Autodesk Inventor part; units mm, degrees
ref_plane "YZ Plane" through (0, 0, 0) normal (1, 0, 0) x (0, 1, 0)
ref_plane "XZ Plane" through (0, 0, 0) normal (0, 1, 0) x (-1, 0, 0)
ref_plane "XY Plane" through (0, 0, 0) normal (0, 0, 1) x (1, 0, 0)
sketch "Sketch1" plane through (0, 0, 0) normal (0, 0, 1) x (1, 0, 0)
  circle A0 centre (0, 0) radius 1.6
  line L0 (9.815, 0) -> (4.9075, -8.5)
  line L1 (4.9075, -8.5) -> (-4.9075, -8.5)
  line L2 (-4.9075, -8.5) -> (-9.815, 0)
  line L3 (-9.815, 0) -> (-4.9075, 8.5)
  line L4 (-4.9075, 8.5) -> (4.9075, 8.5)
  line L5 (4.9075, 8.5) -> (9.815, 0)
  circle A1 centre (0, 0) radius 9.815
  point P0 (-9.815, 0)
  point P1 (-9.815, 0)
  dimension "d0" = 3.2
  dimension "d1" = 17
extrude "Extrusion1" add sketch "Sketch1" along normal blind 4
sketch "Sketch2" plane through (0, 0, 4) normal (0, 0, 1) x (1, 0, 0)
  circle A0 centre (0, 0) radius 8
  dimension "d4" = 16
extrude "Extrusion2" add sketch "Sketch2" along normal blind 2
sketch "Sketch3" plane through (0, 0, 6) normal (0, 0, 1) x (1, 0, 0)
  circle A0 centre (0, 0) radius 6
  dimension "d7" = 12
extrude "Extrusion3" add sketch "Sketch3" along normal blind 6
thread "Thread1"
sketch "Sketch4" plane through (0, 0, 12) normal (0, 0, 1) x (1, 0, 0)
  circle A0 centre (0, 0) radius 6
hole "Hole1" at (0, 0, 12) direction (0, 0, -1) diameter 9 depth 8
fillet "Fillet1" radius 1 2 edges at (4.9075, 8.5, 0) (4.9075, 8.5, 4)
sketch "Sketch5" plane through (0, 0, 0) normal (0, 0, -1) x (-1, 0, 0)
  circle A0 centre (0, 0) radius 1.6
  circle A1 centre (0, 0) radius 9.815
  line L0 (9.815, 0) -> (4.9075, -8.5)
  line L1 (4.9075, -8.5) -> (-4.9075, -8.5)
  line L2 (-4.9075, -8.5) -> (-9.815, 0)
  line L3 (-9.815, 0) -> (-4.9075, 8.5)
  line L4 (-4.9075, 8.5) -> (4.9075, 8.5)
  line L5 (4.9075, 8.5) -> (9.815, 0)
  point P0 (-9.815, 0)
  point P1 (-9.815, 0)
extrude "Extrusion4" cut sketch "Sketch5" against normal blind 5 contours L5 A1 | A1 L0 | L4 A1 | A1 L1 | L3 A1 | A1 L2
properties part number "fix-screw"
Source: CAD feature listing. Evaluate the final solid. Frame: model axes, mm. A direction names the side the tool comes from. Round coordinates to 2 decimals unless told otherwise and drop trailing zeros. Loops run counter-clockwise (first coordinate to the right, second up) from the corner with the lowest first, then second, coordinate; pieces in that order, holes last. Notation, with made-up numbers: M 62.25,53.25 L 79.25,53.25 A24 ccw 79.25,79.25 Z; hole C 71.5,-15 d4. An arc over 180 degrees is marked long. Use a Markdown table: item, result. Add a question column.
1. Cut plane C-C, the plane y = -3.5. Output: boundary loops of the cut face in (x, z).
2. Ray query, line 1 along Y through (x, z) = (0, 3.2); line 2 along Y through (x, z) = (0, 7.5); line 3 along Z through (x, y) = (-3.75, -7). Return the intervals inside material, ascending. Write a range as [from, to].
3. Set-up query: faces 4 (the cylindrical face through (-6, 0, 9)), 5 (the flat face through (7.327, -4.31, 1.972)). Return all of +Z, -Z, +X, -X, +Y, -Y with unobstructed straight access to the full face (end or side cutting, diameter ignored); none if empty.
4. Contact query for flat-ended pins moving along their axis: pin 1 (7 mm diameter, centred on x = -1.5, y = 0, fed in from +Z); pin 2 (6 mm diameter, centred on y = 3.5, z = 6, fed in from -X); pin 3 (1 mm diameter, centred on y = 4.5, z = 5.5, fed in from -X); pin 4 (1 mm diameter, centred on x = -1.5, z = 8.5, fed in from +Y). Output: stop coordinate, or through.
5. Cut plane A-A, the plane x = 0. Output: boundary loops of the cut face in (y, z), and give its area (3 significant figures).
6. Pull-direction query (Y, two-part tool) for faces 1 (the flat face through (-2, 6, 6)), 2 (the flat face through (2, 0, 4)), 3 (the cylindrical face through (-1.73, 7.81, 4.99)); classes: +Y half, -Y half, draft (parallel to the pull), parting line (faces both ways), or undercut.
7. Cut plane D-D, the plane z = 9.75. Output: boundary loops of the cut face in (x, y).
8. Cut plane B-B, the plane z = 3.5. Output: boundary loops of the cut face in (x, y), and give its area (3 significant figures).
Solution:
| question | item | result |
|---|---|---|
| 1 | outline | M -7.79,0 L 7.79,0 L 7.79,4 L 7.19,4 L 7.19,6 L 4.87,6 L 4.87,12 L 2.83,12 L 2.83,4 L -2.83,4 L -2.83,12 L -4.87,12 L -4.87,6 L -7.19,6 L -7.19,4 L -7.79,4 Z |
| 2 | line 1 | y = [-8.5, -1.6], [1.6, 8.5] |
| 2 | line 2 | y = [-6, -4.5], [4.5, 6] |
| 2 | line 3 | z = [0, 6] |
| 3 | face 4 | +Z |
| 3 | face 5 | +Z, -Z, +X, -Y |
| 4 | pin 1 | stops at z = 12 |
| 4 | pin 2 | stops at x = -9.05 |
| 4 | pin 3 | stops at x = -6.93 |
| 4 | pin 4 | stops at y = 5.92 |
| 5 | outline | M -8.5,0 L -1.6,0 L -1.6,4 L -4.5,4 L -4.5,12 L -6,12 L -6,6 L -8,6 L -8,4 L -8.5,4 Z; M 1.6,0 L 8.5,0 L 8.5,4 L 8,4 L 8,6 L 6,6 L 6,12 L 4.5,12 L 4.5,4 L 1.6,4 Z |
| 5 | area | 87.2 mm2 |
| 6 | face 1 | draft |
| 6 | face 2 | undercut |
| 6 | face 3 | parting line |
| 7 | outline | C 0,0 d12; hole C 0,0 d9 |
| 8 | outline | M -9.68,-0.24 L -5.04,-8.26 A9.68 ccw -4.63,-8.5 L 4.63,-8.5 A9.68 ccw 5.04,-8.26 L 9.68,-0.24 A9.68 ccw 9.68,0.24 L 5.04,8.26 A9.68 ccw 4.63,8.5 L -4.63,8.5 A9.68 ccw -5.04,8.26 L -9.68,0.24 A9.68 ccw Z; hole C 0,0 d3.2 |
| 8 | area | 242 mm2 |
